Input: part model. Units: mm. Frame: model coordinates. Face numbers are marked on the shaded views. A direction names the side the tool comes from. Give positions to 0.01 mm unless a question says otherwise; leave off trailing zeros. Order: outer loops, then holes, each group sorted by start corner. A loop starts at its lowest first (then second) coordinate and runs counter-clockwise, first axis right, second up. Notation, with made-up numbers: (-13.75, -25) - (34.25, -25) arc R30 ccw to (34.25, -1) - close; hole circle Ø11 at (-4.75, -38.5). An arc over 180 degrees is marked (long way). Use a Markdown table: item, result.
from build123d import *

# Parameters (mm, degrees)
BOSS_EXTRUDE1_DEPTH     = 5
BOSS_EXTRUDE2_DEPTH     = 75
CUT_EXTRUDE1_DEPTH      = 101
CUT_EXTRUDE1_DEPTH_BACK = 101
SKETCH4_R               = 12.5
CUT_EXTRUDE2_DEPTH      = 101
CUT_EXTRUDE2_DEPTH_BACK = 101


with BuildPart() as part:
    # Sketch1 → Boss-Extrude1 (new body)
    with BuildSketch(Plane(origin=(0, 0, 0), x_dir=(1, 0, 0), z_dir=(0, 1, 0))):
        Polygon((-183.253175473, 100), (-183.253175473, -100), (-75, -37.5), (75, -37.5), (183.253175473, -100), (183.253175473, 100), (75, 37.5), (-75, 37.5), align=None)
    extrude(amount=BOSS_EXTRUDE1_DEPTH)

    # Sketch2 → Boss-Extrude2 (add)
    with BuildSketch(Plane(origin=(0, 5, 0), x_dir=(1, 0, 0), z_dir=(0, 1, 0))):
        Polygon((-183.253175473, -100), (-75, -37.5), (75, -37.5), (183.253175473, -100), (183.253175473, -94.226497308), (76.339745962, -32.5), (-76.339745962, -32.5), (-183.253175473, -94.226497308), align=None)
        Polygon((-183.253175473, 100), (-75, 37.5), (75, 37.5), (183.253175473, 100), (183.253175473, 94.226497308), (76.339745962, 32.5), (-76.339745962, 32.5), (-183.253175473, 94.226497308), align=None)
    extrude(amount=BOSS_EXTRUDE2_DEPTH)

    # Sketch3 → Cut-Extrude1 (cut, two sides)
    with BuildSketch(Plane.XY) as cut_extrude1_sk:
        Polygon((-183.253175473, 0), (-75, 80), (-183.253175473, 80), align=None)
        Polygon((183.253175473, 0), (75, 80), (183.253175473, 80), align=None)
    extrude(amount=CUT_EXTRUDE1_DEPTH, mode=Mode.SUBTRACT)
    extrude(cut_extrude1_sk.sketch, amount=-CUT_EXTRUDE1_DEPTH_BACK, mode=Mode.SUBTRACT)

    # Sketch4 → Cut-Extrude2 (cut, two sides)
    with BuildSketch(Plane.XY) as cut_extrude2_sk:
        with Locations((-37.5, 40)):
            Circle(SKETCH4_R)
        with Locations((37.5, 40)):
            Circle(SKETCH4_R)
    extrude(amount=CUT_EXTRUDE2_DEPTH, mode=Mode.SUBTRACT)
    extrude(cut_extrude2_sk.sketch, amount=-CUT_EXTRUDE2_DEPTH_BACK, mode=Mode.SUBTRACT)


solid = part.part
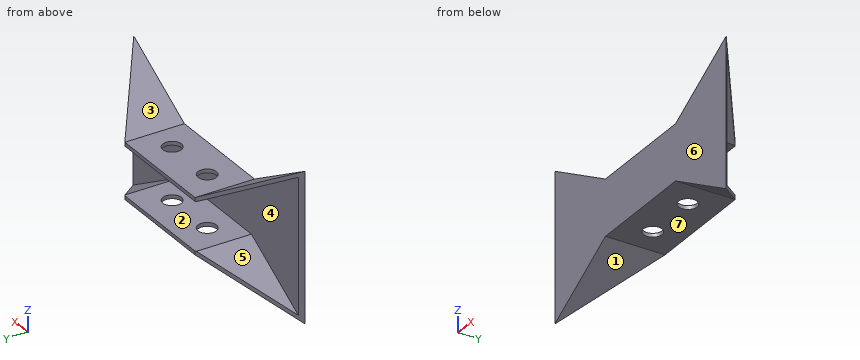
1. Section query B-B (y = 64.5). Return loops of the section in (x, z).
Response:
| item | result |
|---|---|
| outline | (-95.97, -49.61) - (-75, -37.5) - (75, -37.5) - (95.97, -49.61) - (95.97, -43.84) - (76.34, -32.5) - (-76.34, -32.5) - (-95.97, -43.84) - close; (-95.97, 43.84) - (-76.34, 32.5) - (76.34, 32.5) - (95.97, 43.84) - (95.97, 49.61) - (75, 37.5) - (-75, 37.5) - (-95.97, 49.61) - close |
2. Section query A-A (x = 37.5). Return loops of the section in (y, z).
Response:
| item | result |
|---|---|
| outline | (0, -37.5) - (27.5, -37.5) - (27.5, -32.5) - (5, -32.5) - (5, 32.5) - (27.5, 32.5) - (27.5, 37.5) - (0, 37.5) - close; (52.5, -37.5) - (80, -37.5) - (80, -32.5) - (52.5, -32.5) - close; (52.5, 32.5) - (80, 32.5) - (80, 37.5) - (52.5, 37.5) - close |
3. Section query C-C (z = 57). Return loops of the section in (x, y) (3 decimals), then the cut area to 3 significant figures.
Response:
| item | result |
|---|---|
| outline | (-183.253, 0) - (-108.775, 0) - (-108.775, 55.04) - (-118.775, 47.65) - (-118.775, 5) - (-176.487, 5) - close; (108.775, 0) - (183.253, 0) - (176.487, 5) - (118.775, 5) - (118.775, 47.65) - (108.775, 55.04) - close |
| area | 1,640 mm^2 |
4. Pin query (flat end, axial travel): pin 1 (12 mm diameter, centred on y = 58.5, z = -36, fed in from -X); pin 2 (12 mm diameter, centred on x = -129.5, z = 36.5, fed in from +Y); pin 3 (3 mm diameter, centred on x = 0, y = 19, fed in from -Z). Return the tip coordinate at first contact, or that it passes through.
Response:
| item | result |
|---|---|
| pin 1 | stops at x = -92.79 |
| pin 2 | stops at y = 5 |
| pin 3 | stops at z = -37.5 |
5. Material intervals for line 1 along Y through (x, z) = (37.5, 33.55); line 2 along Z through (x, y) = (38, 25.5); line 3 along Y through (x, z) = (-100.5, 16.5), sorted ascending.
Response:
| item | result |
|---|---|
| line 1 | y = 0 to 27.5, 52.5 to 80 |
| line 2 | z = -37.5 to -32.5, 32.5 to 37.5 |
| line 3 | y = 0 to 5 |
6. Section query D-D (y = 40). State how many separate pieces and enclosed holes the cut face has, then the cut area to 3 significant figures.
Response:
| item | result |
|---|---|
| separate pieces | 6 |
| enclosed holes | 0 |
| area | 2,250 mm^2 |
7. Set-up query: the marked faces 1, 2, 3 and 4. Return all of +Z, -Z, +X, -X, +Y, -Y with unobstructed straight access to the full face (end or side cutting, diameter ignored); none if empty.
Response:
| item | result |
|---|---|
| face 1 | -Z, +Y, -Y |
| face 2 | +X, -X, +Y |
| face 3 | +Z, +Y, -Y |
| face 4 | +Y |
8. Mould query, pull axis X, two halves, no side actions, for the marked faces 5, 6 and 7. Classes: pulls with the +X half, pulls with the -X half, needs draft (parallel to the pull), parting line crosses it, or undercut.
Response:
| item | result |
|---|---|
| face 5 | pulls with the -X half |
| face 6 | needs draft |
| face 7 | undercut |
